```python
from build123d import *

# Parameters (mm, degrees)
BOSS_EXTRUDE1_DEPTH      = 30
SHELL1_T                 = -10
BOSS_EXTRUDE2_DEPTH      = 5
BOSS_EXTRUDE2_DEPTH_BACK = 5
BOSS_EXTRUDE3_DEPTH      = 5
BOSS_EXTRUDE3_DEPTH_BACK = 5
BOSS_EXTRUDE4_DEPTH      = 5
BOSS_EXTRUDE4_DEPTH_BACK = 5
BOSS_EXTRUDE5_DEPTH      = 5
BOSS_EXTRUDE5_DEPTH_BACK = 5
BOSS_EXTRUDE6_DEPTH      = 5
BOSS_EXTRUDE6_DEPTH_BACK = 5


with BuildPart() as part:
    # Sketch1 → Boss-Extrude1 (new body)
    with BuildSketch(Plane(origin=(0, 0, 0), x_dir=(1, 0, 0), z_dir=(0, 1, 0))):
        Polygon((-100, -71.262798635), (-100, 71.262798635), (-81.092150171, 169.064846416), (-51.604095563, 203.467576792), (-22.116040956, 219.194539249), (-2.218430034, 219.194539249), (2.218430034, 219.194539249), (22.116040956, 219.194539249), (51.604095563, 203.467576792), (81.092150171, 169.064846416), (100, 71.262798635), (100, -71.262798635), (81.092150171, -169.064846416), (51.604095563, -203.467576792), (22.116040956, -219.194539249), (2.218430034, -219.194539249), (-2.218430034, -219.194539249), (-22.116040956, -219.194539249), (-51.604095563, -203.467576792), (-81.092150171, -169.064846416), align=None)
    extrude(amount=BOSS_EXTRUDE1_DEPTH)

    # Shell1
    shell1_openings = [part.faces().sort_by_distance(p)[0] for p in [
        (0, 30, 0),
    ]]
    offset(amount=SHELL1_T, openings=shell1_openings, kind=Kind.INTERSECTION)

    # Sketch8 → Boss-Extrude2 (add, two sides)
    with BuildSketch(Plane.XY.offset(140)) as boss_extrude2_sk:
        Polygon((-85.23886946, 28.936642873), (-37.764332208, 47), (43.730401993, 46.992588144), (86.132065283, 29.884377125), (76.005879539, 29.884377125), (44.002548329, 42), (-37.120930368, 42), (-74.777956797, 28.936642873), align=None)
    extrude(amount=BOSS_EXTRUDE2_DEPTH)
    extrude(boss_extrude2_sk.sketch, amount=-BOSS_EXTRUDE2_DEPTH_BACK)

    # Sketch4 → Boss-Extrude3 (add, two sides)
    with BuildSketch(Plane.XY.offset(70)) as boss_extrude3_sk:
        Polygon((-100, 30), (-37.764332208, 47), (43.730401993, 46.992588144), (100, 30), (89.335605337, 30), (44.002548329, 42), (-37.120930368, 42), (-90, 30), align=None)
    extrude(amount=BOSS_EXTRUDE3_DEPTH)
    extrude(boss_extrude3_sk.sketch, amount=-BOSS_EXTRUDE3_DEPTH_BACK)

    # Sketch5 → Boss-Extrude4 (add, two sides)
    with BuildSketch(Plane.XY.offset(-70)) as boss_extrude4_sk:
        Polygon((-100, 30), (-37.764332208, 47), (43.730401993, 46.992588144), (100, 30), (89.335605337, 30), (44.002548329, 42), (-37.120930368, 42), (-90, 30), align=None)
    extrude(amount=BOSS_EXTRUDE4_DEPTH)
    extrude(boss_extrude4_sk.sketch, amount=-BOSS_EXTRUDE4_DEPTH_BACK)

    # Sketch7 → Boss-Extrude5 (add, two sides)
    with BuildSketch(Plane.XY.offset(-140)) as boss_extrude5_sk:
        Polygon((86.132065283, 29.884377125), (43.730401993, 46.992588144), (-37.764332208, 47), (-85.23886946, 28.936642873), (-74.777956797, 28.936642873), (-37.120930368, 42), (44.002548329, 42), (76.005879539, 29.884377125), align=None)
    extrude(amount=BOSS_EXTRUDE5_DEPTH)
    extrude(boss_extrude5_sk.sketch, amount=-BOSS_EXTRUDE5_DEPTH_BACK)

    # Sketch2 → Boss-Extrude6 (add, two sides)
    with BuildSketch(Plane.XY) as boss_extrude6_sk:
        Polygon((43.730401993, 46.992588144), (100, 30), (89.335605337, 30), (44.002548329, 42), (-37.120930368, 42), (-90, 30), (-100, 30), (-37.764332208, 47), align=None)
    extrude(amount=BOSS_EXTRUDE6_DEPTH)
    extrude(boss_extrude6_sk.sketch, amount=-BOSS_EXTRUDE6_DEPTH_BACK)


solid = part.part
```
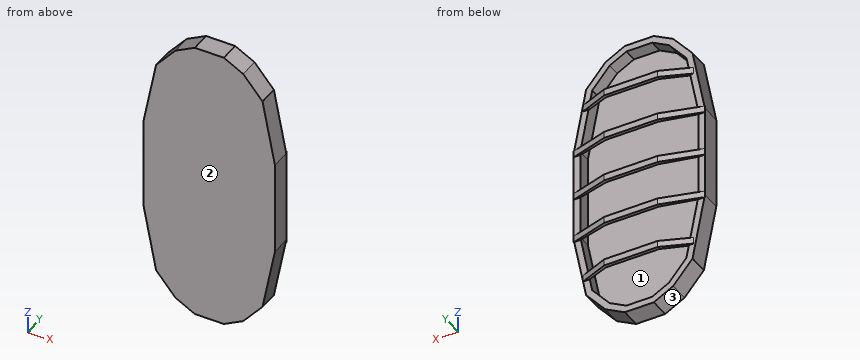
Input: part model. Units: mm. Frame: model coordinates. Face numbers are marked on the shaded views. Coordinates: 2 decimals unless noted, no trailing zeros. Loops run counter-clockwise (first coordinate to the right, second up) from the corner with the lowest first, then second, coordinate; pieces in that order, holes last. Notation, with made-up numbers: M 70,87.5 L 98,87.5 A25 cw 98,110.5 Z; hole C -31,4.5 d1. An arc over 180 degrees is marked long. Answer in a Markdown table with one row per item.
1. Section D-D, the plane x = 7.5. Output: boundary loops of the cut face in (y, z).
Response:
| item | result |
|---|---|
| outline | M 0,-219.19 L 30,-219.19 L 30,-209.19 L 10,-209.19 L 10,209.19 L 30,209.19 L 30,219.19 L 0,219.19 Z; M 42,-145 L 47,-145 L 47,-135 L 42,-135 Z; M 42,-75 L 47,-75 L 47,-65 L 42,-65 Z; M 42,-5 L 47,-5 L 47,5 L 42,5 Z; M 42,65 L 47,65 L 47,75 L 42,75 Z; M 42,135 L 47,135 L 47,145 L 42,145 Z |
2. Material intervals for line 1 (Z direction, x = 26, y = 43); line 2 (Y direction, x = -26.5, z = 2.5); line 3 (X direction, y = 27, z = 46), sorted ascending.
Response:
| item | result |
|---|---|
| line 1 | z = -145 to -135, -75 to -65, -5 to 5, 65 to 75, 135 to 145 |
| line 2 | y = 0 to 10, 42 to 47 |
| line 3 | x = -100 to -90, 90 to 100 |
3. Draft query along X for the marked faces 1, 2 and 3. Return one class per face: pulls with the +X half, pulls with the -X half, needs draft (parallel to the pull), parting line crosses it, or undercut.
Response:
| item | result |
|---|---|
| face 1 | undercut |
| face 2 | needs draft |
| face 3 | pulls with the -X half |
4. First-contact query: pin 1 (1.5 mm diameter, centred on x = -72, z = -54.5, fed in from +Y); pin 2 (12 mm diameter, centred on x = 4.5, z = -73, fed in from +Y); pin 3 (4 mm diameter, centred on y = 7, z = -77, fed in from -X). Flat tips, straight axial feed; report the tip coordinate or a pass-through.
Response:
| item | result |
|---|---|
| pin 1 | stops at y = 10 |
| pin 2 | stops at y = 47 |
| pin 3 | stops at x = -99.28 |
5. Section B-B, the plane x = -30. Output: boundary loops of the cut face in (y, z), then the cut area to 3 significant figures.
Response:
| item | result |
|---|---|
| outline | M 0,-214.99 L 30,-214.99 L 30,-203.66 L 10,-203.66 L 10,203.66 L 30,203.66 L 30,214.99 L 0,214.99 Z; M 42,-145 L 47,-145 L 47,-135 L 42,-135 Z; M 42,-75 L 47,-75 L 47,-65 L 42,-65 Z; M 42,-5 L 47,-5 L 47,5 L 42,5 Z; M 42,65 L 47,65 L 47,75 L 42,75 Z; M 42,135 L 47,135 L 47,145 L 42,145 Z |
| area | 5,000 mm2 |
6. Section C-C, the plane z = -30.5. Output: boundary loops of the cut face in (x, y), then the cut area to 3 significant figures.
Response:
| item | result |
|---|---|
| outline | M -100,0 L 100,0 L 100,30 L 90,30 L 90,10 L -90,10 L -90,30 L -100,30 Z |
| area | 2,400 mm2 |
